Verification items for the finished model (mm, model axes). A direction names the side the tool comes from. Give positions to 0.01 mm unless a question says otherwise; leave off trailing zeros. Loops run counter-clockwise (first coordinate to the right, second up) from the corner with the lowest first, then second, coordinate; pieces in that order, holes last. Notation, with made-up numbers: (-19, -27) - (33, -27) arc R10 ccw to (33, -17) - close; hole circle Ø8 at (75, 68). An arc over 180 degrees is marked (long way). Put each result on its own line as item: value. Start each with the question number.
```python
from build123d import *

# Parameters (mm, degrees)
SKETCH1_W            = 39
SKETCH1_H            = 29
BOSS_EXTRUDE1_DEPTH  = 15
SKETCH2_W            = 37
SKETCH2_H            = 27
CUT_EXTRUDE1_DEPTH   = 14
CHAMFER1_SIZE        = 1
CUT_EXTRUDE2_REACH   = 40.03
SKETCH3_W            = 21
SKETCH3_H            = 5
SKETCH4_W            = 11
SKETCH4_H            = 1
CUT_EXTRUDE3_DEPTH   = 0.5
FILLET1_R            = 0.5
FILLET1_OF_MIRROR2_R = 0.5
SKETCH5_R            = 0.75
BOSS_EXTRUDE2_DEPTH  = 2.5
CHAMFER2_SIZE        = 1


with BuildPart() as part:
    # Sketch1 → Boss-Extrude1 (new body)
    with BuildSketch(Plane(origin=(0, 0, 0), x_dir=(1, 0, 0), z_dir=(0, 1, 0))):
        Rectangle(SKETCH1_W, SKETCH1_H)
    extrude(amount=BOSS_EXTRUDE1_DEPTH)

    # Sketch2 → Cut-Extrude1 (cut)
    with BuildSketch(Plane(origin=(0, 15, 0), x_dir=(1, 0, 0), z_dir=(0, 1, 0))):
        Rectangle(SKETCH2_W, SKETCH2_H)
    extrude(amount=-CUT_EXTRUDE1_DEPTH, mode=Mode.SUBTRACT)

    # Chamfer1
    chamfer1_edges = [part.edges().sort_by_distance(p)[0] for p in [
        (0, 0, 14.5),
        (-19.5, 0, 0),
        (0, 0, -14.5),
        (19.5, 0, 0),
        (19.5, 7.5, 14.5),
        (-19.5, 7.5, 14.5),
        (-19.5, 7.5, -14.5),
        (19.5, 7.5, -14.5),
    ]]
    chamfer(chamfer1_edges, length=CHAMFER1_SIZE)

    # Sketch3 → Cut-Extrude2 (cut, up to next)
    with BuildSketch(Plane.XY.offset(14.5), mode=Mode.PRIVATE) as cut_extrude2_sk1:
        with Locations((0, 7.7)):
            Rectangle(SKETCH3_W, SKETCH3_H)
    cut_extrude2_tool1 = extrude(cut_extrude2_sk1.sketch, amount=-CUT_EXTRUDE2_REACH, mode=Mode.PRIVATE) & part.part
    add(cut_extrude2_tool1.solids().sort_by_distance((0, 7.7, 14.5))[0], mode=Mode.SUBTRACT)

    # Sketch4 → Cut-Extrude3 (cut)
    with BuildSketch(Plane(origin=(-18.5, 0, 0), x_dir=(0, 0, -1), z_dir=(1, 0, 0))):
        with Locations((0, 12.75)):
            Rectangle(SKETCH4_W, SKETCH4_H)
    cut_extrude3 = extrude(amount=-CUT_EXTRUDE3_DEPTH, mode=Mode.SUBTRACT)

    # Fillet1
    fillet1_edges = [part.edges().sort_by_distance(p)[0] for p in [
        (-19, 12.75, 5.5),
    ]]
    fillet(fillet1_edges, radius=FILLET1_R - 0.0001)  # a hair under: the kernel refuses the full size
    fillet1_2_edges = [part.edges().sort_by_distance(p)[0] for p in [
        (-19, 13.25, -0.24995),
    ]]
    fillet(fillet1_2_edges, radius=FILLET1_R - 0.0001)  # a hair under: the kernel refuses the full size
    fillet1_3_edges = [part.edges().sort_by_distance(p)[0] for p in [
        (-19, 12.50005, -5.5),
    ]]
    fillet(fillet1_3_edges, radius=FILLET1_R - 0.0001)  # a hair under: the kernel refuses the full size
    fillet1_4_edges = [part.edges().sort_by_distance(p)[0] for p in [
        (-19, 12.25, 0),
    ]]
    fillet(fillet1_4_edges, radius=FILLET1_R - 0.0001)  # a hair under: the kernel refuses the full size

    # Mirror2: Cut-Extrude3 across plane
    add(cut_extrude3.mirror(Plane(origin=(0, 0, 0), x_dir=(0, 0, 1), z_dir=(1, 0, 0))), mode=Mode.SUBTRACT)

    # Fillet1 of Mirror2
    fillet1_of_mirror2_edges = [part.edges().sort_by_distance(p)[0] for p in [
        (19, 12.25, 0),
    ]]
    fillet(fillet1_of_mirror2_edges, radius=FILLET1_OF_MIRROR2_R - 0.0001)  # a hair under: the kernel refuses the full size
    fillet1_of_mirror2_2_edges = [part.edges().sort_by_distance(p)[0] for p in [
        (19, 12.99995, -5.5),
    ]]
    fillet(fillet1_of_mirror2_2_edges, radius=FILLET1_OF_MIRROR2_R - 0.0001)  # a hair under: the kernel refuses the full size
    fillet1_of_mirror2_3_edges = [part.edges().sort_by_distance(p)[0] for p in [
        (19, 13.25, 0.24995),
    ]]
    fillet(fillet1_of_mirror2_3_edges, radius=FILLET1_OF_MIRROR2_R - 0.0001)  # a hair under: the kernel refuses the full size
    fillet1_of_mirror2_4_edges = [part.edges().sort_by_distance(p)[0] for p in [
        (19, 12.75, 5.5),
    ]]
    fillet(fillet1_of_mirror2_4_edges, radius=FILLET1_OF_MIRROR2_R - 0.0001)  # a hair under: the kernel refuses the full size

    # Sketch5 → Boss-Extrude2 (add)
    # profile 1 of 3: a face of its own
    with BuildSketch(Plane(origin=(0, 1, 0), x_dir=(1, 0, 0), z_dir=(0, 1, 0))):
        with BuildLine():
            Line((-18.5, -13.5), (-12.5, -13.5))
            Line((-12.5, -13.5), (-12.5, -10.5))
            ThreePointArc((-12.5, -10.5), (-13.378679656, -8.378679656), (-15.5, -7.5))
            Line((-15.5, -7.5), (-18.5, -7.5))
            Line((-18.5, -7.5), (-18.5, -13.5))
        make_face()
        with Locations(Location((-14.9, -9.9, 0), (0, 0, 270))):
            Circle(SKETCH5_R, mode=Mode.SUBTRACT)
    # profile 2 of 3: a face of its own
    with BuildSketch(Plane(origin=(0, 1, 0), x_dir=(1, 0, 0), z_dir=(0, 1, 0))):
        with BuildLine():
            Line((-5, 9.5), (5, 9.5))
            ThreePointArc((5, 9.5), (7.5, 7), (5, 4.5))
            Line((5, 4.5), (-5, 4.5))
            ThreePointArc((-5, 4.5), (-7.5, 7), (-5, 9.5))
        make_face()
    # profile 3 of 3: a face of its own
    with BuildSketch(Plane(origin=(0, 1, 0), x_dir=(1, 0, 0), z_dir=(0, 1, 0))):
        with BuildLine():
            Line((12.5, -13.5), (12.5, -10.5))
            ThreePointArc((12.5, -10.5), (13.378679656, -8.378679656), (15.5, -7.5))
            Line((15.5, -7.5), (18.5, -7.5))
            Line((18.5, -7.5), (18.5, -13.5))
            Line((18.5, -13.5), (12.5, -13.5))
        make_face()
        with Locations(Location((14.9, -9.9, 0), (0, 0, 90))):
            Circle(SKETCH5_R, mode=Mode.SUBTRACT)
    extrude(amount=BOSS_EXTRUDE2_DEPTH)

    # Chamfer2
    chamfer2_edges = [part.edges().sort_by_distance(p)[0] for p in [
        (-10.5, 7.7, 14.5),
        (0, 5.2, 14.5),
        (10.5, 7.7, 14.5),
        (0, 10.2, 14.5),
    ]]
    chamfer(chamfer2_edges, length=CHAMFER2_SIZE - 0.0001)  # a hair under: the kernel refuses the full size


solid = part.part
```
1) Set-up check for faces 1 (the face through (11, 8, 14)), 2 (the face through (-18.8, 0.7, -13.9)), 3 (the face through (16, 3.5, 10)): record each of +Z, -Z, +X, -X, +Y, -Y from which the full face is reachable in a straight line by a thin tool's end or side.
2) Scan lines: line 1 along X through (y, z) = (9.5, -12.25); line 2 along X through (y, z) = (2.5, 9.9); line 3 along Z through (x, y) = (17.5, 6.75). Record each from-to range of solid material in increasing order. Write a range as from..to.
3) Section check A-A, the plane y = 2.5. Enter the section's corners in (x, z), plus the area to 3 significant figures.
4) Section check D-D, the plane x = -14.9. Enter the section's corners in (y, z), plus the area to 3 significant figures.
5) Section check B-B, the plane z = -7. Enter the section's corners in (x, y).
6) Draft check along X on faces 4 (the face through (18.9, 0.7, -13.8)), 5 (the face through (-0.2, 10.7, 14)), 6 (the face through (-0.3, 0.5, -14)). Enter one of: pulls with the +X half, pulls with the -X half, needs draft (parallel to the pull), parting line crosses it, or undercut.
7) Depth check by flat-ended pin: P1, Ø1.8, axis at x = -15, z = 10, coming from the +Y side; P2, Ø3, axis at x = 0, z = 1.5, coming from the +Y side. Enter the tip coordinate at first touch or a pass-through.
Results are:
1. face 1: +Z
1. face 2: -Z, -X, -Y
1. face 3: +Y
2. line 1: x = -19.5..-18.5, 18.5..19.5
2. line 2: x = -19.5..-15.65, -14.15..-12.56, 12.56..14.15, 15.65..19.5
2. line 3: z = -14.5..-13.5, 13.5..14.5
3. outline: (-19.5, -13.5) - (-18.5, -14.5) - (18.5, -14.5) - (19.5, -13.5) - (19.5, 13.5) - (18.5, 14.5) - (-18.5, 14.5) - (-19.5, 13.5) - close; (-5, -9.5) - (5, -9.5) arc R2.5 ccw to (5, -4.5) - (-5, -4.5) arc R2.5 ccw to start; hole (-18.5, -13.5) - (18.5, -13.5) - (18.5, 7.5) - (15.5, 7.5) arc R3 cw to (12.5, 10.5) - (12.5, 13.5) - (-12.5, 13.5) - (-12.5, 10.5) arc R3 cw to (-15.5, 7.5) - (-18.5, 7.5) - close; hole circle Ø1.5 at (-14.9, 9.9); hole circle Ø1.5 at (14.9, 9.9)
3. area: 264 mm2
4. outline: (0, -13.5) - (1, -14.5) - (15, -14.5) - (15, -13.5) - (1, -13.5) - (1, 7.56) - (3.5, 7.56) - (3.5, 9.15) - (1, 9.15) - (1, 10.65) - (3.5, 10.65) - (3.5, 13.5) - (15, 13.5) - (15, 14.5) - (1, 14.5) - (0, 13.5) - close
4. area: 67.1 mm2
5. outline: (-19.5, 1) - (-18.5, 0) - (18.5, 0) - (19.5, 1) - (19.5, 15) - (18.5, 15) - (18.5, 1) - (7.5, 1) - (7.5, 3.5) - (-7.5, 3.5) - (-7.5, 1) - (-18.5, 1) - (-18.5, 15) - (-19.5, 15) - close
6. face 4: pulls with the +X half
6. face 5: undercut
6. face 6: needs draft
7. P1: stops at y = 3.5
7. P2: stops at y = 1
